from build123d import *

# Parameters (mm, degrees)
F0_R     = 2.1
F1_DEPTH = 1.6


# Not quite as in the source:
# - a feature names something its author has since deleted; it is built from what else it names


with BuildPart() as f1:
    # F0 (on Top) → F1 (new body)
    with BuildSketch(Plane.XY):
        with BuildLine():
            ThreePointArc((-10, -10), (-2.9289321881, -7.0710678119), (0, 0))
            ThreePointArc((0, 0), (-2.9289321881, 7.0710678119), (-10, 10))
            ThreePointArc((-10, 10), (-20, 0), (-10, -10))
        make_face()
        with Locations((-10, 0)):
            Circle(F0_R, mode=Mode.SUBTRACT)
        with BuildLine():
            ThreePointArc((10, 10), (2.9289321881, 7.0710678119), (0, 0))
            ThreePointArc((0, 0), (2.9289321881, -7.0710678119), (10, -10))
            ThreePointArc((10, -10), (17.0710678119, -7.0710678119), (20, 0))
            ThreePointArc((20, 0), (17.0710678119, 7.0710678119), (10, 10))
        make_face()
        with Locations((10, 0)):
            Circle(F0_R, mode=Mode.SUBTRACT)
        with BuildLine():
            ThreePointArc((-10, 10), (-2.9289321881, 7.0710678119), (0, 0))
            ThreePointArc((0, 0), (2.9289321881, 7.0710678119), (10, 10))
            Line((10, 10), (-10, 10))
        make_face()
        with BuildLine():
            ThreePointArc((10, -10), (2.9289321881, -7.0710678119), (0, 0))
            ThreePointArc((0, 0), (-2.9289321881, -7.0710678119), (-10, -10))
            Line((-10, -10), (10, -10))
        make_face()
    extrude(amount=F1_DEPTH)


solid = f1.part
Design review of the part built by this model. Coordinates are the model's own, in mm. Coordinates: 2 decimals unless noted, no trailing zeros. Loops run counter-clockwise (first coordinate to the right, second up) from the corner with the lowest first, then second, coordinate; pieces in that order, holes last. Notation, with made-up numbers: M 40,27 L 62,27 A19 ccw 62,36 Z; hole C -1.75,56 d11. An arc over 180 degrees is marked long. Use one line per item in the form item = value.
(1) Clearance check with a flat-ended pin moving along its axis: P1, Ø5, axis at x = 10, y = 0, coming from the -Z side. State where the tip first meets the part, or that it passes through.
Return value:
P1 = 0
(2) Consider section B-B (x = -11). Write out the cut boundary in (y, z).
Return value:
outline = M -9.95,0 L -1.85,0 L -1.85,1.6 L -9.95,1.6 Z; M 1.85,0 L 9.95,0 L 9.95,1.6 L 1.85,1.6 Z
(3) For line 1 along X through (y, z) = (-1.5, 1.35); line 2 along X through (y, z) = (-1, 1.5); line 3 along Y through (x, z) = (10, 0.6), list the stretches that pass through material, from the lowest coordinate up. Write a range as from..to.
Return value:
line_1 = -19.89..-11.47, -8.53..8.53, 11.47..19.89
line_2 = -19.95..-11.85, -8.15..8.15, 11.85..19.95
line_3 = -10..-2.1, 2.1..10
(4) Consider section A-A (z = 0.3). Write out the cut boundary in (x, y).
Return value:
outline = M -10,-10 L 10,-10 A10 ccw 10,10 L -10,10 A10 ccw Z; hole C -10,0 d4.2; hole C 10,0 d4.2
(5) Consider section C-C (y = -8). Write out the cut boundary in (x, z), and give its area (3 significant figures).
Return value:
outline = M -16,0 L 16,0 L 16,1.6 L -16,1.6 Z
area = 51.2 mm2
(6) Consider section D-D (x = 14). Write out the cut boundary in (y, z), and give its area (3 significant figures).
Return value:
outline = M -9.17,0 L 9.17,0 L 9.17,1.6 L -9.17,1.6 Z
area = 29.3 mm2
(7) Draft analysis for pull direction Y (two halves, no side actions). For faces 1 (the face through (0, -10, 1)), 2 (the face through (0, 0, 0)), 3 (the face through (-12.1, 0.09, 0.79)), state which applies: pulls with the +Y half, pulls with the -Y half, needs draft (parallel to the pull), parting line crosses it, or undercut.
Return value:
face_1 = pulls with the -Y half
face_2 = needs draft
face_3 = undercut
